from build123d import *

# Parameters (mm, degrees)
BOSS_EXTRUDE1_DEPTH = 584.2
BOSS_EXTRUDE2_START = 584.2
SKETCH2_W           = 31.75
SKETCH2_H           = 31.75
SKETCH2_R           = 5.588
BOSS_EXTRUDE2_DEPTH = 3.175


with BuildPart() as part:
    # Sketch1 → Boss-Extrude1 (new, symmetric)
    with BuildSketch(Plane.XY):
        Polygon((31.75, 1.5875), (1.5875, 1.5875), (1.5875, 31.75), (0, 31.75), (0, 0), (31.75, 0), align=None)
    extrude(amount=BOSS_EXTRUDE1_DEPTH, both=True)

    # Sketch2 → Boss-Extrude2 (add)
    with BuildSketch(Plane.XY.offset(BOSS_EXTRUDE2_START)):
        with Locations((15.875, 15.875)):
            Rectangle(SKETCH2_W, SKETCH2_H)
        with Locations((15.875, 15.875)):
            Circle(SKETCH2_R, mode=Mode.SUBTRACT)
    boss_extrude2 = extrude(amount=-BOSS_EXTRUDE2_DEPTH)

    # Mirror1: Boss-Extrude2 across plane
    add(boss_extrude2.mirror(Plane.XY))


solid = part.part
Can you work these out from the model? Positions are in its coordinate system, mm. A direction names the side the tool comes from. Round coordinates to 2 decimals unless told otherwise and drop trailing zeros. Order: outer loops, then holes, each group sorted by start corner. A loop starts at its lowest first (then second) coordinate and runs counter-clockwise, first axis right, second up. Notation, with made-up numbers: M 61.5,13.5 L 83.5,13.5 A21 cw 83.5,19.5 Z; hole C 40.25,8 d1. An arc over 180 degrees is marked long. Use a Markdown table: item, result.
1) I'm going to push flat-ended pins straight in: P1, Ø9, axis at x = 15.5, y = 16, coming from the -Z side; P2, Ø3, axis at y = 10.5, z = 172, coming from the +X side. Where does each tip first touch, or does it pass through?
Geometry says:
| item | result |
|---|---|
| P1 | passes through |
| P2 | stops at x = 1.59 |
2) Imagine slicing it at A-A (z = -440). List the corners of the cut face in (x, y) for me, then the cut area to 3 significant figures.
Geometry says:
| item | result |
|---|---|
| outline | M 0,0 L 31.75,0 L 31.75,1.59 L 1.59,1.59 L 1.59,31.75 L 0,31.75 Z |
| area | 98.3 mm² |
3) On a 3-axis mill with a long thin cutter (end or side, diameter ignored), from which of +Z, -Z, +X, -X, +Y, -Y can I reach the whole of each face in a straight line? I mean faces 1 (the face through (1.588, 16, 8)), 2 (the face through (1, 31.75, 3)). Say none if no direction works.
Geometry says:
| item | result |
|---|---|
| face 1 | +X, +Y |
| face 2 | +Z, -Z, +X, -X, +Y |
4) If we mould it in two halves opening along Z, with no side actions, what happens to faces 3 (the face through (9, 16, -584.2)), 4 (the face through (20, 20, -581.025)), 5 (the face through (16, 0, 8))? For each: +Z half, -Z half, draft (parallel to the pull), parting line (faces both ways), or undercut.
Geometry says:
| item | result |
|---|---|
| face 3 | -Z half |
| face 4 | undercut |
| face 5 | draft |
5) If I drill on line 1 along Z through (x, y) = (21, 26) (3 decimals); line 2 along Y through (x, z) = (21, -17.5), over which ranges is the centre line in solid material (lowest first)?
Geometry says:
| item | result |
|---|---|
| line 1 | z = -584.2 to -581.025, 581.025 to 584.2 |
| line 2 | y = 0 to 1.59 |
